Read the model definition and answer for the solid it produces. Units are mm, in the model's axes. A direction names the side the tool comes from. Round coordinates to 2 decimals unless told otherwise and drop trailing zeros. Order: outer loops, then holes, each group sorted by start corner. A loop starts at its lowest first (then second) coordinate and runs counter-clockwise, first axis right, second up.
from build123d import *

# Parameters (mm, degrees)
SKETCH1_W           = 110
SKETCH1_H           = 175
SKETCH1_R           = 1.5
BOSS_EXTRUDE1_DEPTH = 12
SKETCH2_W           = 110
SKETCH2_H           = 12
BOSS_EXTRUDE2_DEPTH = 75
SKETCH2_3_W         = 110
SKETCH2_3_H         = 12
BOSS_EXTRUDE3_DEPTH = 60
SKETCH3_R           = 6.5
CUT_EXTRUDE1_DEPTH  = 240.428486192
CUT_EXTRUDE2_REACH  = 241.428
SKETCH3_3_R         = 2.5
SKETCH3_3_R_2       = 20
SKETCH3_4_R         = 5
CUT_EXTRUDE3_DEPTH  = 240.428486192
FILLET1_R           = 10
FILLET2_R           = 15


with BuildPart() as part:
    # Sketch1 → Boss-Extrude1 (new body)
    with BuildSketch(Plane.XY):
        with Locations((55, 87.5)):
            Rectangle(SKETCH1_W, SKETCH1_H)
        with Locations((95, 10)):
            Circle(SKETCH1_R, mode=Mode.SUBTRACT)
        with Locations((75, 10)):
            Circle(SKETCH1_R, mode=Mode.SUBTRACT)
        with Locations(Location((95, 30, 0), (0, 0, 180))):
            Circle(SKETCH1_R, mode=Mode.SUBTRACT)
        with Locations(Location((75, 30, 0), (0, 0, 180))):
            Circle(SKETCH1_R, mode=Mode.SUBTRACT)
        with Locations(Location((35, 10, 0), (0, 0, 180))):
            Circle(SKETCH1_R, mode=Mode.SUBTRACT)
        with Locations(Location((15, 10, 0), (0, 0, 180))):
            Circle(SKETCH1_R, mode=Mode.SUBTRACT)
        with Locations((15, 30)):
            Circle(SKETCH1_R, mode=Mode.SUBTRACT)
        with Locations((35, 30)):
            Circle(SKETCH1_R, mode=Mode.SUBTRACT)
        with Locations(Location((95, 100, 0), (0, 0, 180))):
            Circle(SKETCH1_R, mode=Mode.SUBTRACT)
        with Locations((95, 80)):
            Circle(SKETCH1_R, mode=Mode.SUBTRACT)
        with Locations((75, 80)):
            Circle(SKETCH1_R, mode=Mode.SUBTRACT)
        with Locations(Location((75, 100, 0), (0, 0, 180))):
            Circle(SKETCH1_R, mode=Mode.SUBTRACT)
        with Locations((35, 100)):
            Circle(SKETCH1_R, mode=Mode.SUBTRACT)
        with Locations((15, 100)):
            Circle(SKETCH1_R, mode=Mode.SUBTRACT)
        with Locations(Location((35, 80, 0), (0, 0, 180))):
            Circle(SKETCH1_R, mode=Mode.SUBTRACT)
        with Locations(Location((15, 80, 0), (0, 0, 180))):
            Circle(SKETCH1_R, mode=Mode.SUBTRACT)
    extrude(amount=BOSS_EXTRUDE1_DEPTH)

    # Sketch2 → Boss-Extrude2 (add)
    with BuildSketch(Plane(origin=(0, 0, 0), x_dir=(-1, 0, 0), z_dir=(0, 0, -1))):
        with Locations((-55, 181)):
            Rectangle(SKETCH2_W, SKETCH2_H)
    extrude(amount=-BOSS_EXTRUDE2_DEPTH)

    # Sketch2<3> → Boss-Extrude3 (add)
    with BuildSketch(Plane(origin=(0, 0, 0), x_dir=(-1, 0, 0), z_dir=(0, 0, -1))):
        with Locations((-55, -6)):
            Rectangle(SKETCH2_3_W, SKETCH2_3_H)
    extrude(amount=-BOSS_EXTRUDE3_DEPTH)

    # Sketch3 → Cut-Extrude1 (cut, through all)
    with BuildSketch(Plane(origin=(0, 187, 0), x_dir=(1, 0, 0), z_dir=(0, 1, 0))):
        with Locations(Location((15, -43, 0), (0, 0, 270))):
            Circle(SKETCH3_R)
        with Locations(Location((95, -43, 0), (0, 0, 270))):
            Circle(SKETCH3_R)
    extrude(amount=-CUT_EXTRUDE1_DEPTH, mode=Mode.SUBTRACT)

    # Sketch3<3> → Cut-Extrude2 (cut, up to next)
    with BuildSketch(Plane(origin=(0, 187, 0), x_dir=(1, 0, 0), z_dir=(0, 1, 0)), mode=Mode.PRIVATE) as cut_extrude2_sk1:
        with Locations(Location((31.5, -19.5, 0), (0, 0, 270))):
            Circle(SKETCH3_3_R)
    cut_extrude2_tool1 = extrude(cut_extrude2_sk1.sketch, amount=-CUT_EXTRUDE2_REACH, mode=Mode.PRIVATE) & part.part
    # Sketch3<3> → Cut-Extrude2 (cut, up to next)
    with BuildSketch(Plane(origin=(0, 187, 0), x_dir=(1, 0, 0), z_dir=(0, 1, 0)), mode=Mode.PRIVATE) as cut_extrude2_sk2:
        with Locations(Location((78.5, -19.5, 0), (0, 0, 270))):
            Circle(SKETCH3_3_R)
    cut_extrude2_tool2 = extrude(cut_extrude2_sk2.sketch, amount=-CUT_EXTRUDE2_REACH, mode=Mode.PRIVATE) & part.part
    # Sketch3<3> → Cut-Extrude2 (cut, up to next)
    with BuildSketch(Plane(origin=(0, 187, 0), x_dir=(1, 0, 0), z_dir=(0, 1, 0)), mode=Mode.PRIVATE) as cut_extrude2_sk3:
        with Locations(Location((31.5, -66.5, 0), (0, 0, 270))):
            Circle(SKETCH3_3_R)
    cut_extrude2_tool3 = extrude(cut_extrude2_sk3.sketch, amount=-CUT_EXTRUDE2_REACH, mode=Mode.PRIVATE) & part.part
    # Sketch3<3> → Cut-Extrude2 (cut, up to next)
    with BuildSketch(Plane(origin=(0, 187, 0), x_dir=(1, 0, 0), z_dir=(0, 1, 0)), mode=Mode.PRIVATE) as cut_extrude2_sk4:
        with Locations(Location((78.5, -66.5, 0), (0, 0, 270))):
            Circle(SKETCH3_3_R)
    cut_extrude2_tool4 = extrude(cut_extrude2_sk4.sketch, amount=-CUT_EXTRUDE2_REACH, mode=Mode.PRIVATE) & part.part
    # Sketch3<3> → Cut-Extrude2 (cut, up to next)
    with BuildSketch(Plane(origin=(0, 187, 0), x_dir=(1, 0, 0), z_dir=(0, 1, 0)), mode=Mode.PRIVATE) as cut_extrude2_sk5:
        with Locations(Location((55, -43, 0), (0, 0, 270))):
            Circle(SKETCH3_3_R_2)
    cut_extrude2_tool5 = extrude(cut_extrude2_sk5.sketch, amount=-CUT_EXTRUDE2_REACH, mode=Mode.PRIVATE) & part.part
    add(cut_extrude2_tool1.solids().sort_by_distance((31.5, 187, 19.5))[0], mode=Mode.SUBTRACT)
    add(cut_extrude2_tool2.solids().sort_by_distance((78.5, 187, 19.5))[0], mode=Mode.SUBTRACT)
    add(cut_extrude2_tool3.solids().sort_by_distance((31.5, 187, 66.5))[0], mode=Mode.SUBTRACT)
    add(cut_extrude2_tool4.solids().sort_by_distance((78.5, 187, 66.5))[0], mode=Mode.SUBTRACT)
    add(cut_extrude2_tool5.solids().sort_by_distance((55, 187, 43))[0], mode=Mode.SUBTRACT)

    # Sketch3<4> → Cut-Extrude3 (cut, through all)
    with BuildSketch(Plane(origin=(0, 187, 0), x_dir=(1, 0, 0), z_dir=(0, 1, 0))):
        with Locations(Location((55, -43, 0), (0, 0, 270))):
            Circle(SKETCH3_4_R)
    extrude(amount=-CUT_EXTRUDE3_DEPTH, mode=Mode.SUBTRACT)

    # Fillet1
    # the kernel refuses this fillet: 10 mm, written as the material it adds along each edge
    with BuildSketch(Plane(origin=(110, 175, 12), x_dir=(0, -1, 0), z_dir=(-1, 0, 0))) as fillet1_piece_1_section:
        with BuildLine():
            CenterArc((FILLET1_R, FILLET1_R), FILLET1_R, 180, 90)
            Line((0, FILLET1_R), (-FILLET1_R * 0.02, FILLET1_R))
            Line((-FILLET1_R * 0.02, FILLET1_R), (-FILLET1_R * 0.02, -FILLET1_R * 0.02))
            Line((-FILLET1_R * 0.02, -FILLET1_R * 0.02), (FILLET1_R, -FILLET1_R * 0.02))
            Line((FILLET1_R, -FILLET1_R * 0.02), (FILLET1_R, 0))
        make_face()
    fillet1_piece_1 = extrude(amount=110, mode=Mode.PRIVATE)
    fillet1_piece_1 = fillet1_piece_1 - Plane(origin=(78.5, 172.718411152, 19.5), x_dir=(0, 0, 1), z_dir=(0, 1, 0)) * Cylinder(2.5, 260, mode=Mode.PRIVATE)
    fillet1_piece_1 = fillet1_piece_1 - Plane(origin=(31.5, 172.718411152, 19.5), x_dir=(0, 0, 1), z_dir=(0, 1, 0)) * Cylinder(2.5, 260, mode=Mode.PRIVATE)
    add(fillet1_piece_1)
    with BuildSketch(Plane(origin=(0, 0, 12), x_dir=(0, 1, 0), z_dir=(1, 0, 0))) as fillet1_piece_2_section:
        with BuildLine():
            CenterArc((FILLET1_R, FILLET1_R), FILLET1_R, 180, 90)
            Line((0, FILLET1_R), (-FILLET1_R * 0.02, FILLET1_R))
            Line((-FILLET1_R * 0.02, FILLET1_R), (-FILLET1_R * 0.02, -FILLET1_R * 0.02))
            Line((-FILLET1_R * 0.02, -FILLET1_R * 0.02), (FILLET1_R, -FILLET1_R * 0.02))
            Line((FILLET1_R, -FILLET1_R * 0.02), (FILLET1_R, 0))
        make_face()
    fillet1_piece_2 = extrude(amount=110, mode=Mode.PRIVATE)
    fillet1_piece_2 = fillet1_piece_2 - Plane(origin=(95, 10, 14.266654876), x_dir=(1, 0, 0), z_dir=(0, 0, -1)) * Cylinder(1.5, 260, mode=Mode.PRIVATE)
    fillet1_piece_2 = fillet1_piece_2 - Plane(origin=(75, 10, 14.266654876), x_dir=(1, 0, 0), z_dir=(0, 0, -1)) * Cylinder(1.5, 260, mode=Mode.PRIVATE)
    fillet1_piece_2 = fillet1_piece_2 - Plane(origin=(35, 10, 14.266654876), x_dir=(-1, 0, 0), z_dir=(0, 0, -1)) * Cylinder(1.5, 260, mode=Mode.PRIVATE)
    fillet1_piece_2 = fillet1_piece_2 - Plane(origin=(15, 10, 14.266654876), x_dir=(-1, 0, 0), z_dir=(0, 0, -1)) * Cylinder(1.5, 260, mode=Mode.PRIVATE)
    add(fillet1_piece_2)

    # Fillet2
    fillet2_edges = [part.edges().sort_by_distance(p)[0] for p in [
        (110, 181, 75),
        (0, 181, 75),
        (110, -6, 60),
        (0, -6, 60),
    ]]
    fillet(fillet2_edges, radius=FILLET2_R)


solid = part.part
Q1. For faces 4 (the face through (31.6, 180.4, 17)), 5 (the face through (105.72, -5.92, 55.49)), 6 (the face through (55.77, 172.15, 15.01)), determine the directions among +Z, -Z, +X, -X, +Y, -Y from which every point of the face is accessible in a straight line to the end or side of a thin tool.
Outcome:
face 4: +Y
face 5: +Z, +X, -Y
face 6: +Z, +X, -X
Q2. Flat-ended cylindrical pins translate along their axes: pin 1 (12 mm diameter, centred on x = 56.5, z = 58.5, fed in from +Y); pin 2 (3.5 mm diameter, centred on x = 51.5, y = -8.5, fed in from +Z); pin 3 (3.5 mm diameter, centred on x = 15, y = 10, fed in from +Z); pin 4 (5 mm diameter, centred on x = 35, y = 100, fed in from +Z). Find the tip coordinate at first contact, or state that the pin passes through.
Outcome:
pin 1: stops at y = 187
pin 2: stops at z = 60
pin 3: stops at z = 12.15
pin 4: stops at z = 12
Q3. For a pull along Y with two mould halves and no side action, classify faces 1 (the face through (44, 175, 60)), 2 (the face through (56, -12, 30)), 3 (the face through (105.72, 181.08, 70.49)) as released by +Y, released by -Y, zero draft, split by the parting line, or undercut.
Outcome:
face 1: undercut
face 2: released by -Y
face 3: zero draft
Q4. A cutting plane is placed at B-B, the plane z = 27. Give the vertices of the cut face in (x, y), plus the area to 3 significant figures.
Outcome:
outline: (0, -12) - (110, -12) - (110, 0) - (0, 0) - close; (0, 175) - (43, 175) - (43, 187) - (0, 187) - close; (67, 175) - (110, 175) - (110, 187) - (67, 187) - close
area: 2,350 mm2
Q5. A cutting plane is placed at D-D, the plane x = 70. Give the vertices of the cut face in (y, z), plus the area to 3 significant figures.
Outcome:
outline: (-12, 0) - (187, 0) - (187, 29.77) - (175, 29.77) - (175, 22) arc R10 cw to (165, 12) - (10, 12) arc R10 cw to (0, 22) - (0, 60) - (-12, 60) - close; (175, 56.23) - (187, 56.23) - (187, 75) - (175, 75) - close
area: 3,450 mm2
Q6. A cutting plane is placed at C-C, the plane x = 24.5. Give the vertices of the cut face in (y, z), plus the area to 3 significant figures.
Outcome:
outline: (-12, 0) - (187, 0) - (187, 75) - (175, 75) - (175, 22) arc R10 cw to (165, 12) - (10, 12) arc R10 cw to (0, 22) - (0, 60) - (-12, 60) - close
area: 3,760 mm2
Q7. A cutting plane is placed at A-A, the plane x = 55. Give the vertices of the cut face in (y, z), plus the area to 3 significant figures.
Outcome:
outline: (-12, 0) - (187, 0) - (187, 23) - (175, 23) - (175, 22) arc R10 cw to (165, 12) - (10, 12) arc R10 cw to (0, 22) - (0, 38) - (-12, 38) - close; (-12, 48) - (0, 48) - (0, 60) - (-12, 60) - close; (175, 63) - (187, 63) - (187, 75) - (175, 75) - close
area: 3,160 mm2
Q8. Straight lines are drawn through the part: probe 1 along X at (y, z) = (-9, 43); probe 2 along Y at (x, z) = (75, 4); probe 3 along X at (y, z) = (80, 6.25). For each, find the intervals that lie inside material, in ascending order.
Outcome:
probe 1: x = 0 to 8.5, 21.5 to 50, 60 to 88.5, 101.5 to 110
probe 2: y = -12 to 8.5, 11.5 to 28.5, 31.5 to 78.5, 81.5 to 98.5, 101.5 to 187
probe 3: x = 0 to 13.5, 16.5 to 33.5, 36.5 to 73.5, 76.5 to 93.5, 96.5 to 110
